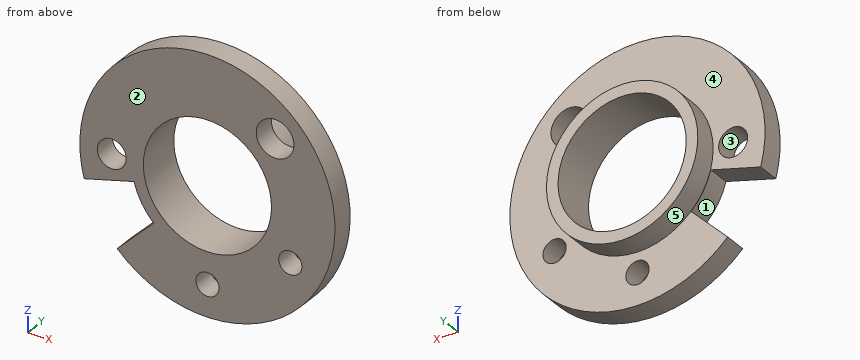
from build123d import *

# Parameters (mm, degrees)
SKETCH3_R          = 2.5
SKETCH3_R_2        = 3.25
SKETCH3_R_3        = 2
CUT_EXTRUDE1_DEPTH = 10


with BuildPart() as part:
    # Sketch1 → Revolve1 (revolve)
    with BuildSketch(Plane.XY, mode=Mode.PRIVATE) as revolve1_sk:
        Polygon((11.05, 0), (11.05, 8), (13.05, 8), (13.05, 3.969255392), (22, 3.969255392), (22, 0), align=None)
    revolve(revolve1_sk.sketch.rotate(Axis((0, 0, 0), (0, 1, 0)), 90), axis=Axis((0, 0, 0), (0, 1, 0)))

    # Sketch3 → Cut-Extrude1 (cut)
    with BuildSketch(Plane(origin=(0, 0, 0), x_dir=(1, 0, 0), z_dir=(0, 1, 0))):
        with Locations(Location((-16.5, 0, 0), (0, 0, 270))):
            Circle(SKETCH3_R)
        with Locations(Location((11.66726189, -11.66726189, 0), (0, 0, 270))):
            Circle(SKETCH3_R_2)
        with Locations(Location((14.289419162, 8.25, 0), (0, 0, 270))):
            Circle(SKETCH3_R_3)
        with Locations(Location((0, 16.5, 0), (0, 0, 270))):
            Circle(SKETCH3_R_3)
        with BuildLine():
            Line((-16.442045207, 16.442045207), (-9.269550975, 9.269550975))
            ThreePointArc((-9.269550975, 9.269550975), (-11.352835017, 6.554562353), (-12.662442113, 3.392891138))
            Line((-12.662442113, 3.392891138), (-22.460251443, 6.018206236))
            ThreePointArc((-22.460251443, 6.018206236), (-20.137310542, 11.626281662), (-16.442045207, 16.442045207))
        make_face()
    extrude(amount=CUT_EXTRUDE1_DEPTH, mode=Mode.SUBTRACT)


solid = part.part
CAD build for the part. Positions are in the model's coordinates, mm. Face numbers are marked on the shaded views. A direction names the side the tool comes from. Coordinates: 2 decimals unless noted, no trailing zeros. Loops run counter-clockwise (first coordinate to the right, second up) from the corner with the lowest first, then second, coordinate; pieces in that order, holes last. Notation, with made-up numbers: (37.5, 75.25) - (50.5, 75.25) arc R17 ccw to (50.5, 90.25) - close; hole circle Ø2 at (-30.75, 78.25). An arc over 180 degrees is marked (long way). Use one line per item in the form item = value. Start each with the question number.
1) Flat gauge pins, fed straight in: pin 1 (1.5 mm diameter, centred on y = 7, z = 6, fed in from +X); pin 2 (3 mm diameter, centred on x = -12, y = 1.5, fed in from -Z); pin 3 (1 mm diameter, centred on y = 7, z = -6, fed in from +X). Where does each tip first touch, or does it go through?
2) Band-saw the part on B-B (z = 0). Give the cut face in (x, y).
3) Two-plate mould, pull along X, no slides. Class the marked faces 3, 4 and 5: +X half, -X half, draft (parallel to the pull), parting line (faces both ways), or undercut.
4) Drill centre lines: L1, parallel to X at y = 3.25, z = -6.5; L2, parallel to X at y = 2, z = -8.25; L3, parallel to Z at x = 2.5, y = 7. Where is each one in solid material? Low to high. Write a range as from..to.
5) Tool access for the marked faces 1 and 2: list every direction of +Z, -Z, +X, -X, +Y, -Y with a clear straight run to the whole face (end or side of a thin tool).
6) Band-saw the part on C-C (y = 1). Give the cut face in (x, z), and give its area (3 significant figures).
7) Band-saw the part on A-A (x = 0). Give the cut face in (y, z), and give its area (3 significant figures).
8) Band-saw the part on D-D (z = -16.5). Give the cut face in (x, y), and give its area (3 significant figures).
Check values:
q1.pin_1 = 11.95
q1.pin_2 = -19.33
q1.pin_3 = 11.83
q2.outline = (-22, 0) - (-19, 0) - (-19, 3.97) - (-22, 3.97) - close; (-14, 0) - (-11.05, 0) - (-11.05, 8) - (-13.05, 8) - (-13.05, 3.97) - (-14, 3.97) - close; (11.05, 0) - (22, 0) - (22, 3.97) - (13.05, 3.97) - (13.05, 8) - (11.05, 8) - close
q3.face_3 = undercut
q3.face_4 = draft
q3.face_5 = parting line
q4.L1 = -11.38..-8.94, 8.94..13.32, 15.26..21.02
q4.L2 = -10.19..-7.35, 7.35..12.29, 16.29..20.39
q4.L3 = -12.81..-10.76, 10.76..12.81
q5.face_1 = +Y, -Y
q5.face_2 = +Z, -Z, +X, -X, -Y
q6.outline = (-21.25, -5.69) - (-12.66, -3.39) arc R13.11 ccw to (-9.27, -9.27) - (-15.56, -15.56) arc R22 ccw (long way) to start; hole circle Ø5 at (-16.5, 0); hole circle Ø22.1 at (0, 0); hole circle Ø4 at (0, -16.5); hole circle Ø6.5 at (11.67, 11.67); hole circle Ø4 at (14.29, -8.25)
q6.area = 977 mm2
q7.outline = (0, -22) - (3.97, -22) - (3.97, -18.5) - (0, -18.5) - close; (0, -14.5) - (3.97, -14.5) - (3.97, -13.05) - (8, -13.05) - (8, -11.05) - (0, -11.05) - close; (0, 11.05) - (8, 11.05) - (8, 13.05) - (3.97, 13.05) - (3.97, 22) - (0, 22) - close
q7.area = 87.2 mm2
q8.outline = (-14.55, 0) - (-2, 0) - (-2, 3.97) - (-14.55, 3.97) - close; (2, 0) - (14.55, 0) - (14.55, 3.97) - (2, 3.97) - close
q8.area = 99.6 mm2
